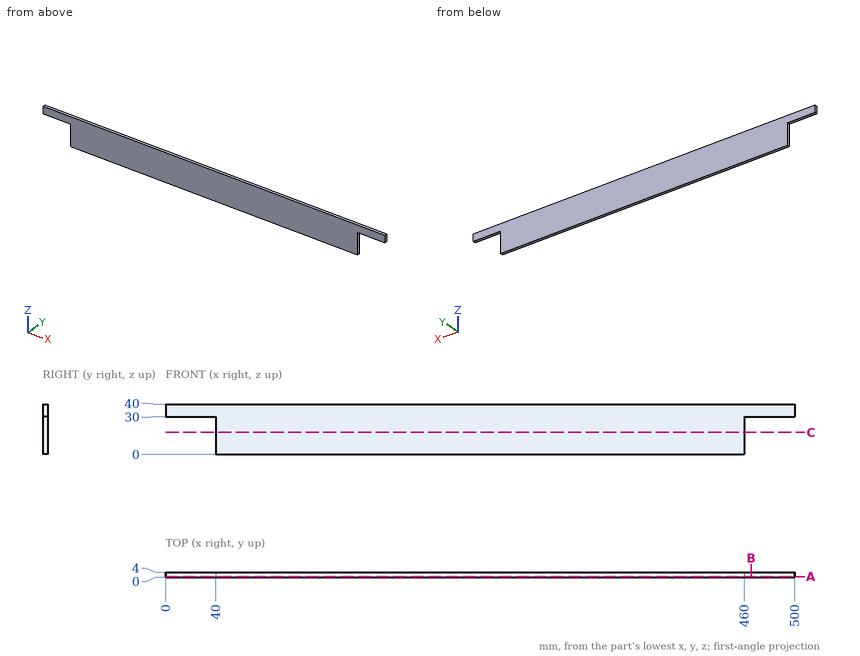
Could you check a few things on this drawing? It's one solid part, dimensions in mm from its lowest x, y, z. Give positions to 0.01 mm unless a question says otherwise; leave off trailing zeros. Order: outer loops, then holes, each group sorted by start corner. A loop starts at its lowest first (then second) coordinate and runs counter-clockwise, first axis right, second up. Notation, with made-up numbers: (43.5, -13) - (50.5, -13) arc R25 cw to (50.5, 4) - close; hole circle Ø10 at (43.25, -19.75). An arc over 180 degrees is marked (long way). One line per question, with ' | ' between items. Start each with the question number.
Item 1: I want a section at C-C on z = 17.5. Write out the boundary of the cut face in (x, y).
Item 2: I'm going to push flat-ended pins straight in: pin 1 Ø2 at (y, z) = (3, 20.5) entering from -X; pin 2 Ø2 at (x, y) = (18, 1.5) entering from -Z. Where does each tip first touch, or does it pass through?
Item 3: I need wall thicknesses on probe 1 along X at (y, z) = (2.05, 24); probe 2 along Z at (x, y) = (30.5, 0.4). Which ranges of each line are inside material? Lowest first, please. Write a range as [from, to].
Item 4: I want a section at A-A on y = 0.6. Write out the boundary of the cut face in (x, z).
Item 5: I want a section at B-B on x = 465.5. Write out the boundary of the cut face in (y, z).
Verdict:
1) outline: (40, 0) - (460, 0) - (460, 4) - (40, 4) - close
2) pin 1: x = 40 | pin 2: z = 30
3) probe 1: [40, 460] | probe 2: [30, 40]
4) outline: (0, 30) - (40, 30) - (40, 0) - (460, 0) - (460, 30) - (500, 30) - (500, 40) - (0, 40) - close
5) outline: (0, 30) - (4, 30) - (4, 40) - (0, 40) - close
